Read the model definition and answer for the solid it produces. Units are mm, in the model's axes. A direction names the side the tool comes from. Coordinates: 2 decimals unless noted, no trailing zeros. Write each loop counter-clockwise with the first axis right and the second up, starting at its lowest first coordinate (ties: lowest second). Pieces come first, ordered by that corner, then holes.
from build123d import *

# Parameters (mm, degrees)
SKETCH1_W      = 42.6
SKETCH1_H      = 42.6
SKETCH1_R      = 1.5
EXTRUDE1_DEPTH = 40.5
EXTRUDE2_DEPTH = 40.5
SKETCH5_R      = 11
EXTRUDE3_DEPTH = 2
SKETCH6_R      = 2.5
EXTRUDE4_DEPTH = 18


with BuildPart() as part:
    # Sketch1 → Extrude1 (new body)
    with BuildSketch(Plane.XY):
        with Locations((21.3, -4.1)):
            Rectangle(SKETCH1_W, SKETCH1_H)
        with Locations((5.8, 11.4)):
            Circle(SKETCH1_R, mode=Mode.SUBTRACT)
        with Locations((5.8, -19.6)):
            Circle(SKETCH1_R, mode=Mode.SUBTRACT)
        with Locations((36.8, -19.6)):
            Circle(SKETCH1_R, mode=Mode.SUBTRACT)
        with Locations((36.8, 11.4)):
            Circle(SKETCH1_R, mode=Mode.SUBTRACT)
    extrude(amount=EXTRUDE1_DEPTH)

    # Sketch2 → Extrude2 (cut)
    with BuildSketch(Plane(origin=(0, 0, 0), x_dir=(-1, 0, 0), z_dir=(0, 0, -1))):
        Polygon((-4.764447963, -25.4), (0, -20.64), (0, -25.4), align=None)
        Polygon((-4.764447963, 17.2), (0, 12.680245569), (0, 17.2), align=None)
        Polygon((-38.128194488, 17.2), (-42.6, 12.680245569), (-42.6, 17.2), align=None)
        Polygon((-38.128194488, -25.4), (-42.6, -20.64), (-42.6, -25.4), align=None)
    extrude(amount=-EXTRUDE2_DEPTH, mode=Mode.SUBTRACT)

    # Sketch5 → Extrude3 (add)
    with BuildSketch(Plane(origin=(0, 0, 0), x_dir=(-1, 0, 0), z_dir=(0, 0, -1))):
        with Locations((-21.3, -4.1)):
            Circle(SKETCH5_R)
    extrude(amount=EXTRUDE3_DEPTH)

    # Sketch6 → Extrude4 (add)
    with BuildSketch(Plane(origin=(0, 0, -2), x_dir=(-1, 0, 0), z_dir=(0, 0, -1))):
        with Locations((-21.3, -4.1)):
            Circle(SKETCH6_R)
    extrude(amount=EXTRUDE4_DEPTH)


solid = part.part
Item 1: The part is cut by section B-B (y = -19.6). Give the vertices of the cut face in (x, z), and give its area (3 significant figures).
Item 2: The part is cut by section A-A (z = 20.5). Give the vertices of the cut face in (x, y), and give its area (3 significant figures).
Item 3: Determine the mould class of faces 1 (the flat face through (2.416, 14.972, 19.966)), 2 (the cylindrical face through (4.3, 11.47, 19.97)), 3 (the flat face through (21, -4, -20)) for opening direction Y: +Y half, -Y half, draft (parallel to the pull), parting line (faces both ways), or undercut.
Item 4: The part is cut by section D-D (y = -4.1). Give the vertices of the cut face in (x, z).
Item 5: The part is cut by section C-C (x = 5.8). Give the vertices of the cut face in (y, z), and give its area (3 significant figures).
Item 6: Given pin 1 (12 mm diameter, centred on y = -3, z = -11.5, fed in from -X); pin 2 (13 mm diameter, centred on x = 11.5, y = -10.5, fed in from -Z); pin 3 (1.5 mm diameter, centred on x = 31.5, y = 9.5, fed in from -Z), each flat-ended and moving along its own axis, determine where each tip first touches the part or whether it passes through.
Item 7: For faces 4 (the cylindrical face through (11.139, -8.313, -0.986)), 5 (the cylindrical face through (4.69, -18.59, 19.97)), determine the directions among +Z, -Z, +X, -X, +Y, -Y from which every point of the face is accessible in a straight line to the end or side of a thin tool.
Item 8: Find the intervals of material crossed by probe 1 along Y at (x, z) = (5.8, 18); probe 2 along Y at (x, z) = (5, 12.5); probe 3 along Z at (x, y) = (20, 15.5), in increasing order.
Answer:
1. outline: (0, 0) - (4.3, 0) - (4.3, 40.5) - (0, 40.5) - close; (7.3, 0) - (35.3, 0) - (35.3, 40.5) - (7.3, 40.5) - close; (38.3, 0) - (42.6, 0) - (42.6, 40.5) - (38.3, 40.5) - close
1. area: 1,480 mm2
2. outline: (0, -20.64) - (4.76, -25.4) - (38.13, -25.4) - (42.6, -20.64) - (42.6, 12.68) - (38.13, 17.2) - (4.76, 17.2) - (0, 12.68) - close; hole circle Ø3 at (5.8, -19.6); hole circle Ø3 at (5.8, 11.4); hole circle Ø3 at (36.8, -19.6); hole circle Ø3 at (36.8, 11.4)
2. area: 1,740 mm2
3. face 1: +Y half
3. face 2: undercut
3. face 3: draft
4. outline: (0, 0) - (10.3, 0) - (10.3, -2) - (18.8, -2) - (18.8, -20) - (23.8, -20) - (23.8, -2) - (32.3, -2) - (32.3, 0) - (42.6, 0) - (42.6, 40.5) - (0, 40.5) - close
5. outline: (-25.4, 0) - (-21.1, 0) - (-21.1, 40.5) - (-25.4, 40.5) - close; (-18.1, 0) - (9.9, 0) - (9.9, 40.5) - (-18.1, 40.5) - close; (12.9, 0) - (17.2, 0) - (17.2, 40.5) - (12.9, 40.5) - close
5. area: 1,480 mm2
6. pin 1: stops at x = 18.8
6. pin 2: stops at z = -2
6. pin 3: stops at z = 0
7. face 4: -Z
7. face 5: +Z, -Z
8. probe 1: y = -25.4 to -21.1, -18.1 to 9.9, 12.9 to 17.2
8. probe 2: y = -25.4 to -20.87, -18.33 to 10.13, 12.67 to 17.2
8. probe 3: z = 0 to 40.5
